For this review, take the finished solid that the model builds, in its own axes (mm). Give positions to 0.01 mm unless a question says otherwise; leave off trailing zeros. Loops run counter-clockwise (first coordinate to the right, second up) from the corner with the lowest first, then second, coordinate; pieces in that order, holes last. Notation, with made-up numbers: (40.25, 25) -> (75.25, 25) arc R20 ccw to (75.25, 44) -> close; hole circle Ø7 at (74.25, 73.25). An arc over 180 degrees is marked (long way). Write each question's results on one line, items separated by ' | '. Start each with the question number.
```python
from build123d import *

# Parameters (mm, degrees)
F1_DEPTH = 50.8
F3_DEPTH = 50.801
F4_W     = 50.8
F4_H     = 6.35
F5_DEPTH = 38.1
F6_R     = 1.5875
F7_DEPTH = 50.801


with BuildPart() as f1:
    # F0 (on Front) → F1 (new body)
    with BuildSketch(Plane.XZ):
        with BuildLine():
            Line((0, 6.35), (0, 0))
            Line((0, 0), (25.4, 0))
            ThreePointArc((25.4, 0), (56.830896, -13.019104), (69.85, -44.45))
            Line((69.85, -44.45), (76.2, -44.45))
            ThreePointArc((76.2, -44.45), (61.321024, -8.528976), (25.4, 6.35))
            Line((25.4, 6.35), (0, 6.35))
        make_face()
    extrude(amount=F1_DEPTH)

    # F2 (on face) → F3 (cut, through all)
    with BuildSketch(Plane.XY.offset(6.35)):
        with BuildLine():
            ThreePointArc((76.2, -28.575), (36.401015, -33.862407), (0, -50.8))
            Line((0, -50.8), (76.2, -50.8))
            Line((76.2, -50.8), (76.2, -28.575))
        make_face()
        with BuildLine():
            Line((76.2, 0), (0, 0))
            ThreePointArc((0, 0), (36.401015, -16.937593), (76.2, -22.225))
            Line((76.2, -22.225), (76.2, 0))
        make_face()
    extrude(amount=-F3_DEPTH, mode=Mode.SUBTRACT)

    # F4 (on face) → F5 (join)
    with BuildSketch(Plane(origin=(0, 0, 0), x_dir=(0, -1, 0), z_dir=(-1, 0, 0))):
        with Locations((25.4, 3.175)):
            Rectangle(F4_W, F4_H)
    extrude(amount=F5_DEPTH)

    # F6 (on face) → F7 (cut, through all)
    with BuildSketch(Plane.XZ.offset(50.8)):
        with Locations((-3.175, 3.175)):
            Circle(F6_R)
    extrude(amount=-F7_DEPTH, mode=Mode.SUBTRACT)


solid = f1.part
```
1. We need section C-C (z = -31). Write out the cut boundary in (x, y), plus the area to 3 significant figures.
2. Draft analysis for pull direction X (two halves, no side actions). For faces 1 (the flat face through (-38.1, -25, 3)), 2 (the flat face through (-6, -25, 0)), 3 (the cylindrical face through (-2.3, -25.8, 4.5)), state which applies: released by +X, released by -X, zero draft, split by the parting line, or undercut.
3. Wall thickness on L1, parallel to Z at x = -8, y = -14; L2, parallel to X at y = -26, z = 1: over which ranges is each line inside the solid? List them lowest first.
4. For pin 1 Ø5 at (x, z) = (-3.175, 3.175) entering from +Y; pin 2 Ø12 at (y, z) = (-24, -3.5) entering from +X; pin 3 Ø3 at (x, y) = (-12, -24) entering from -Z, all flat-tipped, find the tip position at first contact; note any pin that passes through.
5. We need section B-B (x = -25.5). Write out the cut boundary in (y, z).
Response:
1) outline: (67.77, -28.68) arc R132.83 cw to (74.39, -28.55) -> (74.39, -22.25) arc R132.83 cw to (67.77, -22.12) -> close | area: 42.2 mm2
2) face 1: released by -X | face 2: zero draft | face 3: undercut
3) L1: z = 0 to 6.35 | L2: x = -38.1 to 48.09
4) pin 1: stops at y = 0 | pin 2: stops at x = 62.27 | pin 3: stops at z = 0
5) outline: (-50.8, 0) -> (0, 0) -> (0, 6.35) -> (-50.8, 6.35) -> close
